from build123d import *

# Parameters (mm, degrees)
SKETCH_2_R      = 7
SKETCH_2_R_2    = 2.4
EXTRUDE_1_DEPTH = 7.5
SKETCH_4_R      = 2
EXTRUDE_3_DEPTH = 1.25
SKETCH_5_R      = 2.5
SKETCH_5_R_2    = 2
EXTRUDE_4_DEPTH = 5
CHAMFER_1_SIZE  = 1.25


with BuildPart() as part:
    # 草图1 → 旋转1 (revolve)
    with BuildSketch(Plane(origin=(0, -42.25, 0), x_dir=(1, 0, 0), z_dir=(0, 1, 0)), mode=Mode.PRIVATE) as revolve_1_sk:
        Polygon((53.274875926, 15.125), (53.274875926, 17.125), (43.5, 17.125), (43.5, 13.85), (46.25, 13.85), (46.25, 14.725), (49.5, 14.725), (49.5, 13.5), (50.75, 13.5), (50.75, 15.125), align=None)
    revolve(revolve_1_sk.sketch.rotate(Axis((58.375, -42.25, -17.125), (-1, 0, 0)), 180), axis=Axis((58.375, -42.25, -17.125), (-1, 0, 0)))

    # 草图2 → 凸台-拉伸1 (add)
    with BuildSketch(Plane(origin=(0, -46, 0), x_dir=(1, 0, 0), z_dir=(0, 1, 0))):
        with Locations(Location((58.375, 17.125, 0), (0, 0, 270))):
            Circle(SKETCH_2_R)
        with Locations(Location((58.375, 17.125, 0), (0, 0, 270))):
            Circle(SKETCH_2_R_2, mode=Mode.SUBTRACT)
    extrude(amount=EXTRUDE_1_DEPTH)

    # 草图4 → 凸台-拉伸3 (add)
    with BuildSketch(Plane.ZY.offset(-43.5)):
        with Locations(Location((-17.125, -42.25, 0), (0, 0, 180))):
            Circle(SKETCH_4_R)
    extrude(amount=EXTRUDE_3_DEPTH)

    # 草图5 → 凸台-拉伸4 (add)
    # profile 1 of 2: a face of its own
    with BuildSketch(Plane.ZY.offset(-42.25)):
        with Locations((-17.125, -42.25)):
            Circle(SKETCH_5_R)
        with Locations(Location((-17.125, -42.25, 0), (0, 0, 180))):
            Circle(SKETCH_5_R_2, mode=Mode.SUBTRACT)
    # profile 2 of 2: a face of its own
    with BuildSketch(Plane.ZY.offset(-42.25)):
        with Locations(Location((-17.125, -42.25, 0), (0, 0, 180))):
            Circle(SKETCH_5_R_2)
    extrude(amount=EXTRUDE_4_DEPTH)

    # 倒角1
    chamfer_1_edges = [part.edges().sort_by_distance(p)[0] for p in [
        (43.5, -42.25, -13.85),
    ]]
    chamfer(chamfer_1_edges, length=CHAMFER_1_SIZE)


solid = part.part
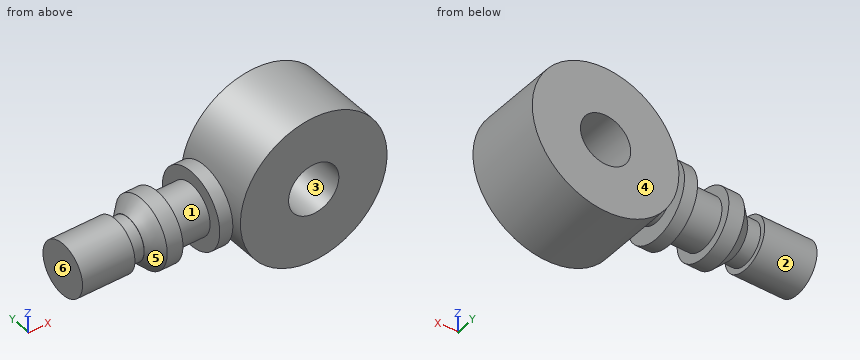
Could you check a few things on this model? Use its own coordinates, in mm. Face numbers are marked on the shaded views. A direction names the side the tool comes from. Round coordinates to 2 decimals unless told otherwise and drop trailing zeros. Order: outer loops, then holes, each group sorted by start corner. A loop starts at its lowest first (then second) coordinate and runs counter-clockwise, first axis right, second up.
Q1. I'm going to push flat-ended pins straight in: P1, Ø1.5, axis at x = 50, y = -45, coming from the -Z side; P2, Ø1.5, axis at y = -42.5, z = -17.5, coming from the +X side (3 decimals); P3, Ø6, axis at x = 43, z = -16, coming from the -Y side (3 decimals); P4, Ø1.5, axis at x = 44.5, y = -45, coming from the -Z side. Where does each tip first touch, or does it pass through?
Geometry says:
P1: stops at z = -20.15
P2: stops at x = 65.375
P3: stops at y = -45.525
P4: stops at z = -19.68
Q2. Which directions (+Z, -Z, +X, -X, +Y, -Y) give clear straight access to the entire face, cutting with the end or side of a thin tool? Please do the marked faces 1, 2 and 3.
Geometry says:
face 1: none
face 2: -X
face 3: +Y, -Y
Q3. Thinking about a two-plate mould opening in X: for the marked faces 4, 5 and 6, which applies, released by +X, released by -X, zero draft, split by the parting line, or undercut?
Geometry says:
face 4: zero draft
face 5: undercut
face 6: released by -X
Q4. Please list where these lines run through material, in increasing order: probe 1 along Z at (x, y) = (58.5, -44.75); probe 2 along X at (y, z) = (-43.5, -15.5); probe 3 along X at (y, z) = (-43.25, -18.5).
Geometry says:
probe 1: z = -24.12 to -19.52, -14.73 to -10.13
probe 2: x = 37.25 to 42.25, 43.53 to 50.75, 51.57 to 56.61, 60.14 to 65.18
probe 3: x = 37.25 to 56.41, 60.34 to 65.24
Q5. Imagine slicing it at B-B, the plane x = 56.25. List the corners of the cut face in (y, z) for me, then the cut area to 3 significant figures.
Geometry says:
outline: (-46, -23.79) - (-38.5, -23.79) - (-38.5, -18.24) - (-46, -18.24) - close; (-46, -16.01) - (-38.5, -16.01) - (-38.5, -10.46) - (-46, -10.46) - close
area: 83.3 mm2
Q6. Imagine slicing it at A-A, the plane y = -42.25. List the corners of the cut face in (x, z) for me (3 decimals).
Geometry says:
outline: (37.25, -19.625) - (42.25, -19.625) - (42.25, -19.125) - (43.5, -19.125) - (43.5, -19.15) - (44.75, -20.4) - (46.25, -20.4) - (46.25, -19.525) - (49.5, -19.525) - (49.5, -20.75) - (50.75, -20.75) - (50.75, -19.125) - (51.667, -19.125) arc R7 ccw (long way) to (51.667, -15.125) - (50.75, -15.125) - (50.75, -13.5) - (49.5, -13.5) - (49.5, -14.725) - (46.25, -14.725) - (46.25, -13.85) - (44.75, -13.85) - (43.5, -15.1) - (43.5, -15.125) - (42.25, -15.125) - (42.25, -14.625) - (37.25, -14.625) - close; hole circle Ø4.8 at (58.375, -17.125)
Q7. Imagine slicing it at C-C, the plane x = 47.25. List the corners of the cut face in (y, z) for me (3 decimals), then the cut area to 3 significant figures.
Geometry says:
outline: circle Ø4.8 at (-42.25, -17.125)
area: 18.1 mm2
Q8. Imagine slicing it at D-D, the plane z = -22. List the corners of the cut face in (x, y) for me.
Geometry says:
outline: (53.35, -46) - (63.4, -46) - (63.4, -38.5) - (53.35, -38.5) - close
